CAD build for the part. Positions are in the model's coordinates, mm. A direction names the side the tool comes from. Coordinates: 2 decimals unless noted, no trailing zeros. Order: outer loops, then holes, each group sorted by start corner. A loop starts at its lowest first (then second) coordinate and runs counter-clockwise, first axis right, second up. Notation, with made-up numbers: (-2, -15.5) -> (13, -15.5) arc R33 ccw to (13, 23.5) -> close; hole circle Ø10 at (41.25, 76). An arc over 180 degrees is marked (long way). Use one line per item in the form item = value. Start each with the question number.
from build123d import *

# Parameters (mm, degrees)
HOLE_WIZARD_M10_1_D     = 8.5
HOLE_WIZARD_M10_1_DEPTH = 24.5
HOLE_WIZARD_M10_1_TIP   = 2.553657631
CHAMFER_1_SIZE          = 1


with BuildPart() as part:
    # 草图1 → 旋转1 (revolve)
    with BuildSketch(Plane.XY):
        with BuildLine():
            Line((0, 0), (8.5, 0))
            Line((8.5, 0), (8.5, 1.8))
            Line((8.5, 1.8), (6.5, 1.8))
            Line((6.5, 1.8), (6.5, 4.8))
            ThreePointArc((6.5, 4.8), (7.999862618, 7.426786408), (6.45, 10.024385409))
            Line((6.45, 10.024385409), (6.45, 18.3))
            Line((6.45, 18.3), (0, 18.3))
            Line((0, 18.3), (0, 0))
        make_face()
    revolve(axis=Axis((0, 0, 0), (0, 1, 0)))

    # M10 螺纹孔1
    with Locations(Plane(origin=(0, 0, 0), x_dir=(-1, 0, 0), z_dir=(0, -1, 0))):
        with Locations((0, 0)):
            Hole(HOLE_WIZARD_M10_1_D / 2, depth=HOLE_WIZARD_M10_1_DEPTH)
            with Locations((0, 0, -(HOLE_WIZARD_M10_1_DEPTH + HOLE_WIZARD_M10_1_TIP / 2))):  # 118° drill point
                Cone(0, HOLE_WIZARD_M10_1_D / 2, HOLE_WIZARD_M10_1_TIP, mode=Mode.SUBTRACT)

    # 倒角1
    chamfer_1_edges = [part.edges().sort_by_distance(p)[0] for p in [
        (-6.45, 18.3, 0),
    ]]
    chamfer(chamfer_1_edges, length=CHAMFER_1_SIZE)


solid = part.part
1) Drop flat-ended pins along their axis: P1, Ø10, axis at x = -5, y = 11, coming from the -Z side; P2, Ø6, axis at x = -3.5, y = 9, coming from the +Z side; P3, Ø5, axis at x = -5, y = 10, coming from the -Z side. Give the stop position or say it passes through.
2) Probe L1, parallel to Z at x = 0, y = 12.75; L2, parallel to Y at x = 4.75, z = -7; L3, parallel to Z at x = 0, y = 7. List the from-to ranges inside material, lowest first.
3) Two-plate mould, pull along Y, no slides. Class faces 1 (the face through (-5.158, 3.321, 3.955)), 2 (the face through (-2, 0, -4)), 3 (the face through (-2, 18.3, 4)): released by +Y, released by -Y, zero draft, split by the parting line, or undercut.
4) Cut at B-B on x = 0. Give the cut face in (y, z), then the cut area to 3 significant figures.
5) Cut at D-D on y = 4. Give the cut face in (x, z).
6) Cut at A-A on z = 0. Give the cut face in (x, y), then the cut area to 3 significant figures.
7) Cut at C-C on y = 15.75. Give the cut face in (x, z).
8) 3-axis set-ups, long thin cutter, end or side, ignore diameter. For faces 4 (the face through (4.4, 1.8, 5)), 5 (the face through (4.57, 0.913, -7.167)), 6 (the face through (-1.398, 13.713, 6.297)): which of +Z, -Z, +X, -X, +Y, -Y reach the whole face in a straight line?
Values follow:
q1.P1 = -7.89
q1.P2 = 7.95
q1.P3 = -7.2
q2.L1 = -6.45 to -4.25, 4.25 to 6.45
q2.L2 = 0 to 1.8
q2.L3 = -7.97 to -4.25, 4.25 to 7.97
q3.face_1 = undercut
q3.face_2 = released by -Y
q3.face_3 = released by +Y
q4.outline = (0, -8.5) -> (1.8, -8.5) -> (1.8, -6.5) -> (4.8, -6.5) arc R3 ccw to (10.02, -6.45) -> (17.3, -6.45) -> (18.3, -5.45) -> (18.3, -4.25) -> (0, -4.25) -> close; (0, 4.25) -> (18.3, 4.25) -> (18.3, 5.45) -> (17.3, 6.45) -> (10.02, 6.45) arc R3 ccw to (4.8, 6.5) -> (1.8, 6.5) -> (1.8, 8.5) -> (0, 8.5) -> close
q4.area = 98.8 mm^2
q5.outline = circle Ø13 at (0, 0); hole circle Ø8.5 at (0, 0)
q6.outline = (-8.5, 0) -> (-4.25, 0) -> (-4.25, 18.3) -> (-5.45, 18.3) -> (-6.45, 17.3) -> (-6.45, 10.02) arc R3 ccw to (-6.5, 4.8) -> (-6.5, 1.8) -> (-8.5, 1.8) -> close; (4.25, 0) -> (8.5, 0) -> (8.5, 1.8) -> (6.5, 1.8) -> (6.5, 4.8) arc R3 ccw to (6.45, 10.02) -> (6.45, 17.3) -> (5.45, 18.3) -> (4.25, 18.3) -> close
q6.area = 98.8 mm^2
q7.outline = circle Ø12.9 at (0, 0); hole circle Ø8.5 at (0, 0)
q8.face_4 = none
q8.face_5 = +Y, -Y
q8.face_6 = +Y
